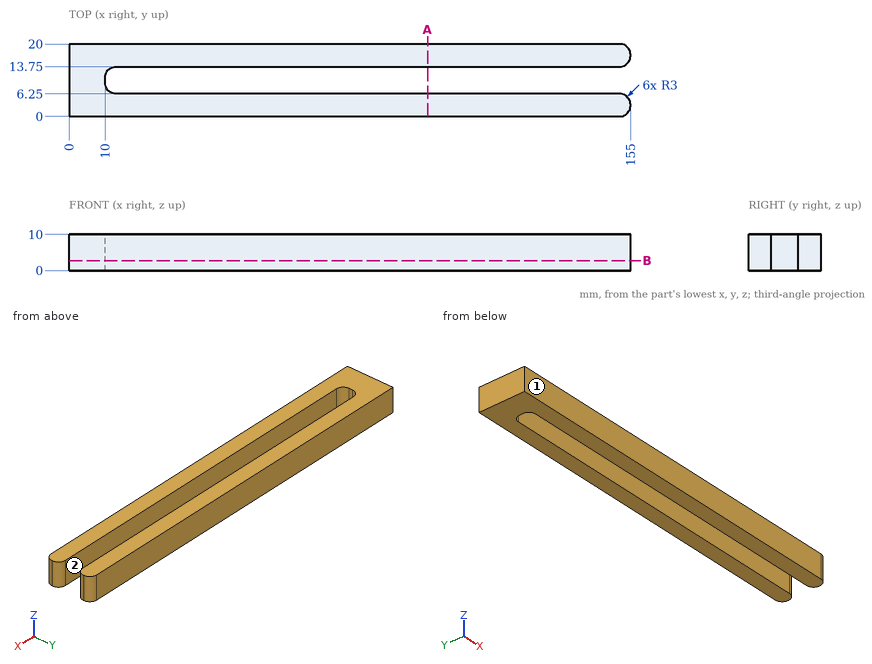
Could you check a few things on this drawing? It's one solid part, dimensions in mm from its lowest x, y, z. A direction names the side the tool comes from. Give positions to 0.01 mm unless a question says otherwise; leave off trailing zeros. Loops run counter-clockwise (first coordinate to the right, second up) from the corner with the lowest first, then second, coordinate; pieces in that order, holes last. Notation, with made-up numbers: (65.25, 21.25) -> (116.25, 21.25) arc R25 cw to (116.25, 50.25) -> close; hole circle Ø4 at (30.5, 43). An arc over 180 degrees is marked (long way). Use one line per item in the form item = value. Start each with the question number.
1) Which directions (+Z, -Z, +X, -X, +Y, -Y) give clear straight access to the entire face, cutting with the end or side of a thin tool? Please do the marked faces 1 and 2.
2) Imagine slicing it at A-A (x = 99). Please give me the cut outline in (y, z), then the cut area to 3 significant figures.
3) Please list where these lines run through material, in increasing order: line 1 along Y through (x, z) = (125, 6); line 2 along X through (y, z) = (9.25, 0.5).
4) For P1, Ø1, axis at y = 10.5, z = 3, coming from the +X side; P2, Ø1.5, axis at y = 5, z = 7, coming from the +X side, each with a flat end and sliding along its axis, tell me the tip position at first contact or that it passes through.
5) Imagine slicing it at B-B (z = 2.75). Please give me the cut outline in (x, y), then the cut area to 3 significant figures.
Check values:
q1.face_1 = +Z, -Z, +X, -X, -Y
q1.face_2 = +Z, -Z, +X
q2.outline = (0, 0) -> (6.25, 0) -> (6.25, 10) -> (0, 10) -> close; (13.75, 0) -> (20, 0) -> (20, 10) -> (13.75, 10) -> close
q2.area = 125 mm^2
q3.line_1 = 0 to 6.25, 13.75 to 20
q3.line_2 = 0 to 10
q4.P1 = 10.01
q4.P2 = 154.83
q5.outline = (0, 0) -> (152, 0) arc R3 ccw to (155, 3) -> (155, 3.25) arc R3 ccw to (152, 6.25) -> (13, 6.25) arc R3 cw to (10, 9.25) -> (10, 10.75) arc R3 cw to (13, 13.75) -> (152, 13.75) arc R3 ccw to (155, 16.75) -> (155, 17) arc R3 ccw to (152, 20) -> (0, 20) -> close
q5.area = 2,010 mm^2
